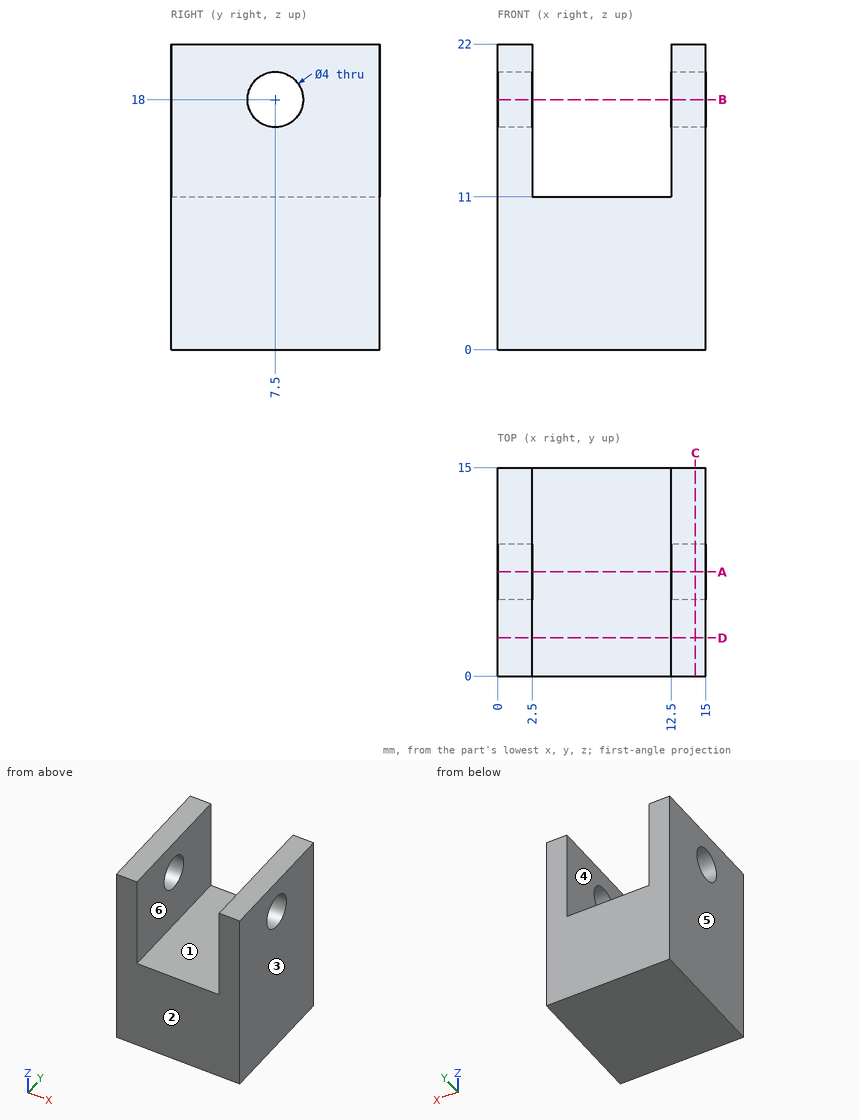
Source: three-view drawing plus pictorial views. Frame: mm from the lowest corner of the part. A direction names the side the tool comes from. Round coordinates to 2 decimals unless told otherwise and drop trailing zeros. Write each loop counter-clockwise with the first axis right and the second up, starting at its lowest first coordinate (ties: lowest second). Pieces come first, ordered by that corner, then holes. Notation, with made-up numbers: M -5,2.25 L 33,2.25 A14 ccw 33,13.25 Z; hole C -5,-6 d9. An arc over 180 degrees is marked long. Use CSV: the item, a comma, the result in double quotes. Start each with the question number.
Q1. Cut plane B-B on z = 18. Output: boundary loops of the cut face in (x, y).
Q2. Cut plane D-D on y = 2.75. Output: boundary loops of the cut face in (x, z), plus the area to 3 significant figures.
Q3. Cut plane A-A on y = 7.5. Output: boundary loops of the cut face in (x, z), plus the area to 3 significant figures.
Q4. Line query: line 1 (X direction, y = 4, z = 15.75); line 2 (Y direction, x = 14.2, z = 18); line 3 (Z direction, x = 9, y = 3.25). Output: solid intervals per line, ascending. Write a range as from..to.
Q5. Cut plane C-C on x = 14.25. Output: boundary loops of the cut face in (y, z).
Q6. First-contact query: P1, Ø8, axis at x = 7, y = 10, coming from the +Z side. Flat tip, straight axial feed; report the tip coordinate or a pass-through.
Q7. Pull-direction query (X, two-part tool) for the marked faces 1, 2, 3 and 4; classes: +X half, -X half, draft (parallel to the pull), parting line (faces both ways), or undercut.
Q8. Access query for the marked faces 5 and 6. Directions: +Z, -Z, +X, -X, +Y, -Y. A direction counts if a zero-diameter tool reaches every point of the face in a straight line with its end or side. Return the directions, or none.
Results found:
1,outline,"M 0,0 L 2.5,0 L 2.5,5.5 L 0,5.5 Z; M 0,9.5 L 2.5,9.5 L 2.5,15 L 0,15 Z; M 12.5,0 L 15,0 L 15,5.5 L 12.5,5.5 Z; M 12.5,9.5 L 15,9.5 L 15,15 L 12.5,15 Z"
2,outline,"M 0,0 L 15,0 L 15,22 L 12.5,22 L 12.5,11 L 2.5,11 L 2.5,22 L 0,22 Z"
2,area,"220 mm^2"
3,outline,"M 0,0 L 15,0 L 15,16 L 12.5,16 L 12.5,11 L 2.5,11 L 2.5,16 L 0,16 Z; M 0,20 L 2.5,20 L 2.5,22 L 0,22 Z; M 12.5,20 L 15,20 L 15,22 L 12.5,22 Z"
3,area,"200 mm^2"
4,line 1,"0..2.5, 12.5..15"
4,line 2,"0..5.5, 9.5..15"
4,line 3,"0..11"
5,outline,"M 0,0 L 15,0 L 15,22 L 0,22 Z; hole C 7.5,18 d4"
6,P1,"z = 11"
7,face 1,"undercut"
7,face 2,"draft"
7,face 3,"+X half"
7,face 4,"undercut"
8,face 5,"+Z, -Z, -X, +Y, -Y"
8,face 6,"+Z, +Y, -Y"
